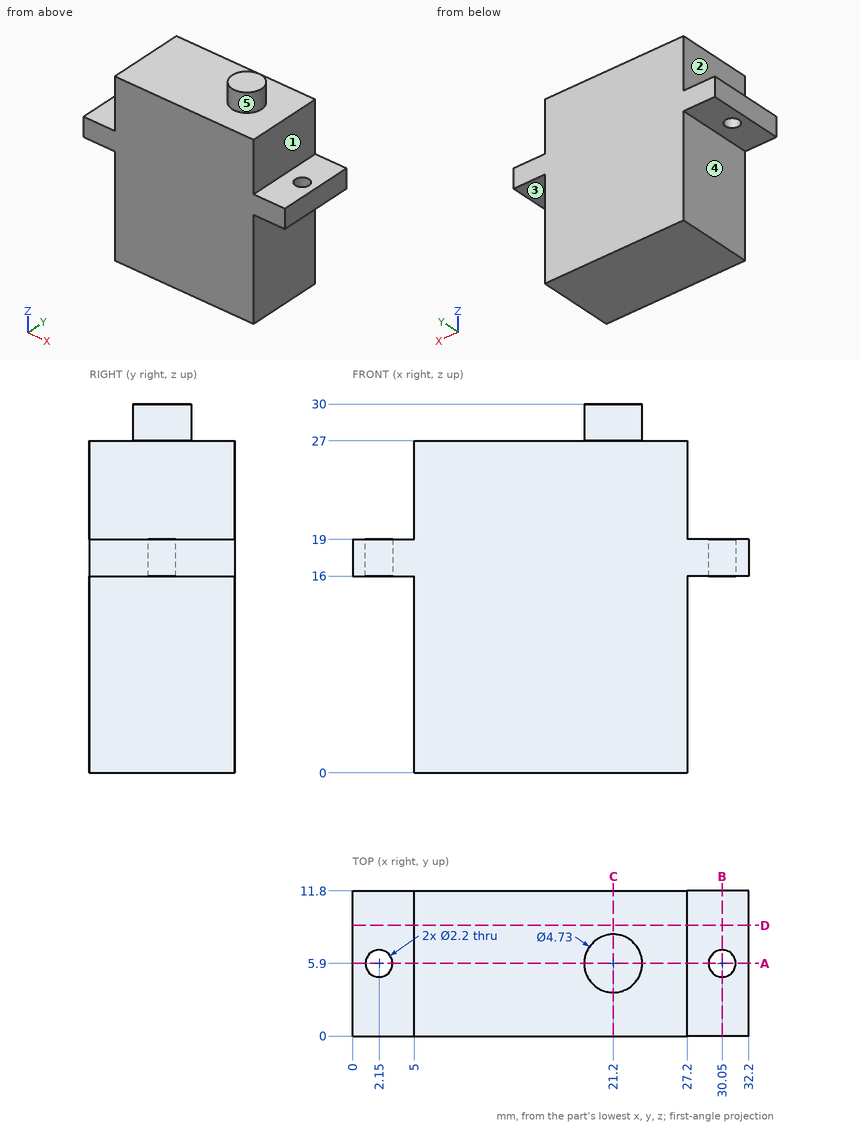
Can you work these out from the drawing? Everything is in mm from the part's minimum corner. A direction names the side the tool comes from. Give positions to 0.01 mm unless a question says otherwise; leave off trailing zeros. Loops run counter-clockwise (first coordinate to the right, second up) from the corner with the lowest first, then second, coordinate; pieces in that order, holes last. Notation, with made-up numbers: (82, -33) -> (95, -33) arc R13 cw to (95, -24) -> close; hole circle Ø9 at (60.5, 16). An arc over 180 degrees is marked (long way). Return JSON: item names as keys, results as strings.
Item 1: If we section it at D-D on y = 9: List the corners of the cut face in (x, z) for me.
Geometry results:
{"outline": "(0, 16) -> (5, 16) -> (5, 0) -> (27.2, 0) -> (27.2, 16) -> (32.2, 16) -> (32.2, 19) -> (27.2, 19) -> (27.2, 27) -> (5, 27) -> (5, 19) -> (0, 19) -> close"}
Item 2: If we section it at C-C on x = 21.2: List the corners of the cut face in (y, z) for me (3 decimals), plus the area to 3 significant figures.
Geometry results:
{"outline": "(0, 0) -> (11.8, 0) -> (11.8, 27) -> (8.265, 27) -> (8.265, 30) -> (3.535, 30) -> (3.535, 27) -> (0, 27) -> close", "area": "333 mm²"}
Item 3: If we section it at B-B on x = 30.05: List the corners of the cut face in (y, z) for me.
Geometry results:
{"outline": "(0, 16) -> (4.8, 16) -> (4.8, 19) -> (0, 19) -> close; (7, 16) -> (11.8, 16) -> (11.8, 19) -> (7, 19) -> close"}
Item 4: If we section it at A-A on y = 5.9: List the corners of the cut face in (x, z) for me (3 decimals), plus the area to 3 significant figures.
Geometry results:
{"outline": "(0, 16) -> (1.05, 16) -> (1.05, 19) -> (0, 19) -> close; (3.25, 16) -> (5, 16) -> (5, 0) -> (27.2, 0) -> (27.2, 16) -> (28.95, 16) -> (28.95, 19) -> (27.2, 19) -> (27.2, 27) -> (23.565, 27) -> (23.565, 30) -> (18.835, 30) -> (18.835, 27) -> (5, 27) -> (5, 19) -> (3.25, 19) -> close; (31.15, 16) -> (32.2, 16) -> (32.2, 19) -> (31.15, 19) -> close", "area": "630 mm²"}
Item 5: Which directions (+Z, -Z, +X, -X, +Y, -Y) give clear straight access to the entire face, cutting with the end or side of a thin tool? Please do the marked faces 1, 2, 3, 4 and 5.
Geometry results:
{"face 1": "+Z, +X, +Y, -Y", "face 2": "+Z, -X, +Y, -Y", "face 3": "-Z, +X, +Y, -Y", "face 4": "-Z, -X, +Y, -Y", "face 5": "+Z"}
Item 6: I'm going to push flat-ended pins straight in: pin 1 (5.5 mm diameter, centred on x = 2, y = 4.5, fed in from +Z); pin 2 (2 mm diameter, centred on y = 8, z = 21.5, fed in from -X); pin 3 (2.5 mm diameter, centred on x = 3, y = 8.5, fed in from -Z); pin 4 (4 mm diameter, centred on x = 18, z = 11, fed in from -Y). Where does each tip first touch, or does it pass through?
Geometry results:
{"pin 1": "stops at z = 19", "pin 2": "stops at x = 5", "pin 3": "stops at z = 16", "pin 4": "stops at y = 0"}
Item 7: I need wall thicknesses on L1, parallel to X at y = 9.75, z = 9; L2, parallel to Z at x = 11, y = 5.5; L3, parallel to Z at x = 30, y = 8.25. Which ranges of each line are inside material? Lowest first, please. Write a range as from..to.
Geometry results:
{"L1": "x = 5..27.2", "L2": "z = 0..27", "L3": "z = 16..19"}
